from build123d import *

# Parameters (mm, degrees)
SKETCH_1_W          = 15
SKETCH_1_H          = 42
EXTRUDE_1_DEPTH     = 3
SKETCH_3_R          = 1.5
SKETCH_3_R_2        = 3
CUT_EXTRUDE_1_DEPTH = 23.5
FILLET_1_R          = 7.5


with BuildPart() as part:
    # 草图1 → 凸台-拉伸1 (new body)
    with BuildSketch(Plane.XY):
        Rectangle(SKETCH_1_W, SKETCH_1_H)
    extrude(amount=EXTRUDE_1_DEPTH)

    # 草图3 → 切除-拉伸1 (cut, through all)
    with BuildSketch(Plane.XY.offset(3)):
        with Locations((0, 16.5)):
            Circle(SKETCH_3_R)
        with Locations((0, 6.5)):
            Circle(SKETCH_3_R)
        with Locations((0, -13.5)):
            Circle(SKETCH_3_R_2)
    extrude(amount=-CUT_EXTRUDE_1_DEPTH, mode=Mode.SUBTRACT)

    # 圆角1
    fillet_1_edges = [part.edges().sort_by_distance(p)[0] for p in [
        (-7.5, -21, 1.5),
        (7.5, -21, 1.5),
    ]]
    fillet(fillet_1_edges, radius=FILLET_1_R - 0.0001)  # a hair under: the kernel refuses the full size


solid = part.part
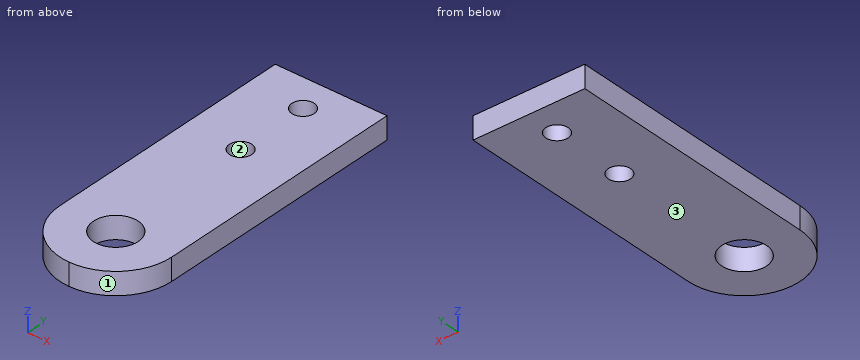
Geometry: final body of the model. Coordinates: model frame, mm. Face numbers are marked on the shaded views. Give positions to 0.01 mm unless a question says otherwise; leave off trailing zeros. Write each loop counter-clockwise with the first axis right and the second up, starting at its lowest first coordinate (ties: lowest second). Pieces come first, ordered by that corner, then holes.
(1) Cut plane A-A, the plane y = 6.5. Return loops of the section in (x, z), then the cut area to 3 significant figures.
(2) Ray query, line 1 (Y direction, x = 0, z = 1.5); line 2 (X direction, y = -15, z = 2.2); line 3 (Y direction, x = -2.25, z = 0.5). Return the intervals inside material, ascending.
(3) Cut plane D-D, the plane x = 5.75. Return loops of the section in (y, z), then the cut area to 3 significant figures.
(4) Mould query, pull axis X, two halves, no side actions, for the marked faces 1, 2 and 3. Classes: released by +X, released by -X, zero draft, split by the parting line, or undercut.
(5) Cut plane B-B, the plane z = 2.3. Give the number of separate pieces and of enclosed holes in the cut face, then the cut area to 3 significant figures.
(6) Cut plane C-C, the plane x = -2.5. Return loops of the section in (y, z), then the cut area to 3 significant figures.
Values follow:
1. outline: (-7.5, 0) - (-1.5, 0) - (-1.5, 3) - (-7.5, 3) - close; (1.5, 0) - (7.5, 0) - (7.5, 3) - (1.5, 3) - close
1. area: 36.0 mm2
2. line 1: y = -21 to -16.5, -10.5 to 5, 8 to 15, 18 to 21
2. line 2: x = -7.35 to -2.6, 2.6 to 7.35
2. line 3: y = -20.65 to -15.48, -11.52 to 21
3. outline: (-18.32, 0) - (21, 0) - (21, 3) - (-18.32, 3) - close
3. area: 118 mm2
4. face 1: released by +X
4. face 2: undercut
4. face 3: zero draft
5. separate pieces: 1
5. enclosed holes: 3
5. area: 563 mm2
6. outline: (-20.57, 0) - (-15.16, 0) - (-15.16, 3) - (-20.57, 3) - close; (-11.84, 0) - (21, 0) - (21, 3) - (-11.84, 3) - close
6. area: 115 mm2
